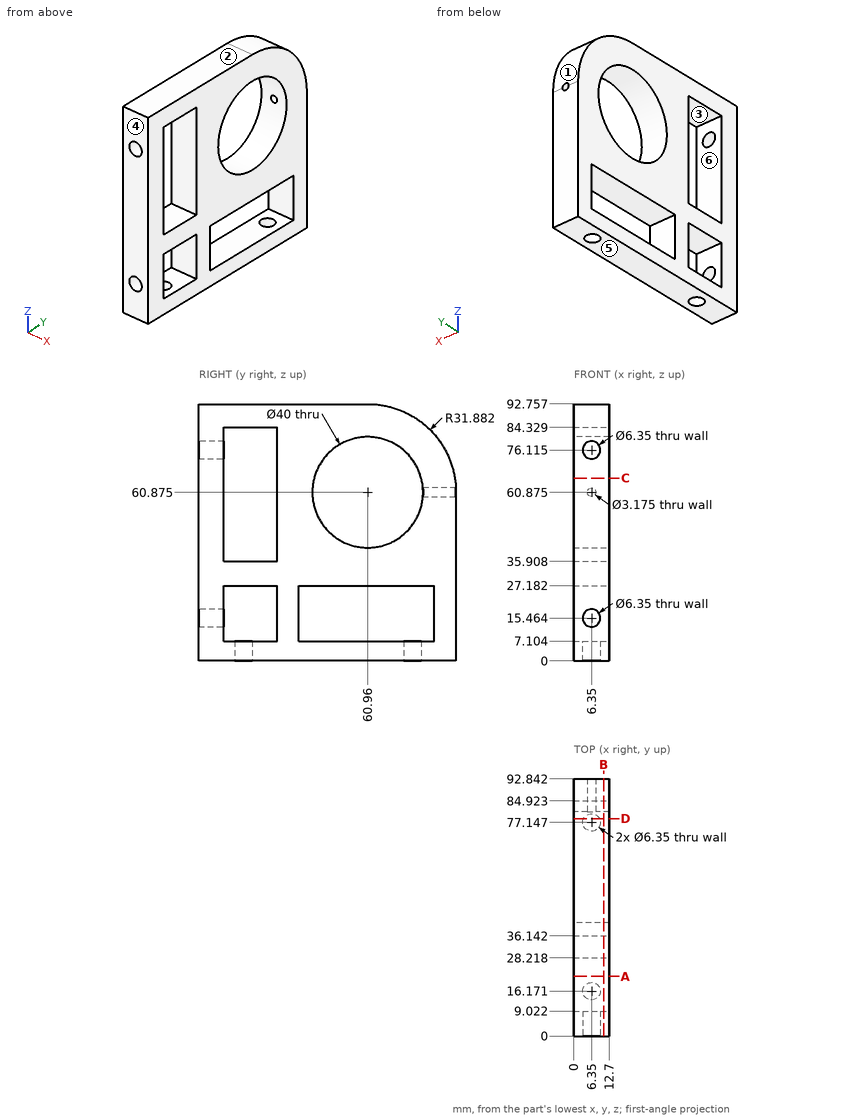
The figure shows three views and two pictorial views of one solid part (mm, origin at its lowest corner). Answer the questions. A direction names the side the tool comes from. Coordinates: 2 decimals unless noted, no trailing zeros. Write each loop counter-clockwise with the first axis right and the second up, starting at its lowest first coordinate (ties: lowest second). Pieces come first, ordered by that corner, then holes. Notation, with made-up numbers: M 75,27.5 L 110,27.5 A24 ccw 110,57.5 Z; hole C -18,58 d11. An arc over 180 degrees is marked long. Answer as CSV lines item,"result". Start each with the question number.
Item 1: Flat-ended cylindrical pins translate along their axes: P1, Ø4, axis at x = 8, z = 64.5, coming from the +Y side; P2, Ø5.5, axis at x = 6.35, y = 77.15, coming from the -Z side. Find the tip coordinate at first contact, or state that the pin passes through.
Item 2: A tool of negligible diameter and unlimited length cuts with its end or side. For the marked faces 5 and 6, from which of +Z, -Z, +X, -X, +Y, -Y can it reach the whole face along a straight path? Write none if from no direction.
Item 3: Section A-A on y = 21.5 is taken. Write down the section's boundary in (x, z), and give its area (3 significant figures).
Item 4: Determine the mould class of the marked faces 1, 2, 3 and 4 for opening direction Y: released by +Y, released by -Y, zero draft, split by the parting line, or undercut.
Item 5: Section B-B on x = 10.75 is taken. Write down the section's boundary in (y, z) (1 decimal).
Item 6: Consider L1, parallel to Z at x = 4.5, y = 12; L2, parallel to Y at x = 2.5, z = 10; L3, parallel to Y at x = 6.35, z = 1.75. Determine where each line is inside the solid, lowest interval first.
Item 7: Section D-D on y = 78.5 is taken. Write down the section's boundary in (x, z) (1 decimal).
Item 8: Section C-C on z = 66 is taken. Write down the section's boundary in (x, y), and give its area (3 significant figures).
Checks:
1,P1,"stops at y = 92.8"
1,P2,"stops at z = 27.18"
2,face 5,"-Z, +X, -X, +Y, -Y"
2,face 6,"+X, -X"
3,outline,"M 0,0 L 12.7,0 L 12.7,7.1 L 0,7.1 Z; M 0,27.18 L 12.7,27.18 L 12.7,35.91 L 0,35.91 Z; M 0,84.33 L 12.7,84.33 L 12.7,92.76 L 0,92.76 Z"
3,area,"308 mm²"
4,face 1,"released by +Y"
4,face 2,"zero draft"
4,face 3,"undercut"
4,face 4,"released by -Y"
5,outline,"M 0,0 L 92.8,0 L 92.8,60.9 A31.9 ccw 61,92.8 L 0,92.8 Z; hole M 9,7.1 L 28.2,7.1 L 28.2,27.2 L 9,27.2 Z; hole M 9,35.9 L 28.2,35.9 L 28.2,84.3 L 9,84.3 Z; hole M 36.1,7.1 L 84.9,7.1 L 84.9,27.2 L 36.1,27.2 Z; hole C 61,60.9 d40"
6,L1,"z = 0 to 7.1, 27.18 to 35.91, 84.33 to 92.76"
6,L2,"y = 0 to 9.02, 28.22 to 36.14, 84.92 to 92.84"
6,L3,"y = 0 to 13, 19.35 to 73.97, 80.32 to 92.84"
7,outline,"M 0,0 L 3.5,0 L 3.5,7.1 L 0,7.1 Z; M 0,27.2 L 12.7,27.2 L 12.7,51.3 L 0,51.3 Z; M 0,70.5 L 12.7,70.5 L 12.7,87.5 L 0,87.5 Z; M 9.2,0 L 12.7,0 L 12.7,7.1 L 9.2,7.1 Z"
8,outline,"M 0,0 L 12.7,0 L 12.7,9.02 L 0,9.02 Z; M 0,28.22 L 12.7,28.22 L 12.7,41.63 L 0,41.63 Z; M 0,80.29 L 12.7,80.29 L 12.7,92.43 L 0,92.43 Z"
8,area,"439 mm²"
